The model under review builds one solid part; all positions refer to its coordinate system, in mm. Coordinates: 2 decimals unless noted, no trailing zeros. Order: outer loops, then holes, each group sorted by start corner. A loop starts at its lowest first (then second) coordinate and runs counter-clockwise, first axis right, second up. Notation, with made-up numbers: M 9,40 L 16,40 A28 cw 16,65 Z; hole C -8.5,28 d6. An arc over 180 degrees is marked long. Write each question's results on one line, items separated by ' | '.
Autodesk Inventor part; units mm, degrees
ref_plane "YZ Plane" through (0, 0, 0) normal (1, 0, 0) x (0, 1, 0)
ref_plane "XZ Plane" through (0, 0, 0) normal (0, 1, 0) x (-1, 0, 0)
ref_plane "XY Plane" through (0, 0, 0) normal (0, 0, 1) x (1, 0, 0)
sketch "Sketch1" plane through (0, 0, 0) normal (0, 0, 1) x (1, 0, 0)
  line L0 (-25.4, 25.4) -> (25.4, 25.4)
  line L1 (25.4, 25.4) -> (25.4, -25.4)
  line L2 (25.4, -25.4) -> (-25.4, -25.4)
  line L3 (-25.4, -25.4) -> (-25.4, 25.4)
  point P0 (0, 0)
  dimension "d0" = 25.4
  dimension "d1" = 50.8
  dimension "d2" = 50.8
  dimension "d3" = 25.4
extrude "Extrusion1" add sketch "Sketch1" along normal blind 2
fillet "Fillet1" radius 3.175 4 edges at (25.4, 25.4, 1) (25.4, -25.4, 1) (-25.4, 25.4, 1) (-25.4, -25.4, 1)
sketch "Sketch2" plane through (0, 0, 2) normal (0, 0, 1) x (1, 0, 0)
  circle A0 centre (-22.4, -0.0994) radius 1.5
  circle A1 centre (11.4, -19.4) radius 1.5
  circle A2 centre (11.4, 19.4) radius 1.5
  line L0 (-25.4, 22.225) -> (-25.4, -22.225)
  line L1 (22.225, 25.4) -> (-22.225, 25.4)
  line L2 (-22.225, -25.4) -> (22.225, -25.4)
  line L3 (25.4, -22.225) -> (25.4, 22.225)
  point P0 (0, 0)
  dimension "d7" = 3
  dimension "d9" = 3
  dimension "d17" = 3
  dimension "d18" = 6
  dimension "d19" = 6
  dimension "d20" = 14
  dimension "d21" = 14
  dimension "d22" = 3
extrude "Extrusion2" cut sketch "Sketch2" against normal blind 2
equation "\"d9\" = d7"
equation "\"d19\" = d18"
equation "\"d21\" = d20"
equation "\"d22\" = d7"
properties part number "breadbord_2_inch"
1) Take a section at A-A on y = -19.4. State the section outline as (x, z) points, plus the area to 3 significant figures.
Solutions:
outline: M -25.4,0 L 9.9,0 L 9.9,2 L -25.4,2 Z; M 12.9,0 L 25.4,0 L 25.4,2 L 12.9,2 Z | area: 95.6 mm2
2) The part is to be moulded in two halves that separate along Y. For faces 1 (the cylindrical face through (-24.45, 24.49, 1.01)), 2 (the flat face through (0, -25.4, 1)), 3 (the cylindrical face through (10.29, -18.39, 1.01)), say which applies: pulls with the +Y half, pulls with the -Y half, needs draft (parallel to the pull), parting line crosses it, or undercut.
Solutions:
face 1: pulls with the +Y half | face 2: pulls with the -Y half | face 3: undercut
3) To check wall thickness, follow line 1 along Y through (x, z) = (11.4, 1.1); line 2 along Y through (x, z) = (-22.4, 1); line 3 along X through (y, z) = (0.5, 0.55). State the ranges of each line that lie inside material, in increasing order.
Solutions:
line 1: -25.4 to -20.9, -17.9 to 17.9, 20.9 to 25.4 | line 2: -25.4 to -1.6, 1.4 to 25.4 | line 3: -25.4 to -23.78, -21.02 to 25.4
4) Take a section at B-B on x = 11.4. State the section outline as (y, z) points, plus the area to 3 significant figures.
Solutions:
outline: M -25.4,0 L -20.9,0 L -20.9,2 L -25.4,2 Z; M -17.9,0 L 17.9,0 L 17.9,2 L -17.9,2 Z; M 20.9,0 L 25.4,0 L 25.4,2 L 20.9,2 Z | area: 89.6 mm2
5) For pin 1 (5 mm diameter, centred on x = 11.4, y = -19.4, fed in from -Z), flat-tipped, find the tip position at first contact; note if it passes through.
Solutions:
pin 1: z = 0
